The listing builds one solid part. Answer for the finished solid, in the listing's coordinates (mm). A direction names the side the tool comes from. Give positions to 0.01 mm unless a question says otherwise; leave off trailing zeros. Write each loop counter-clockwise with the first axis right and the second up, starting at its lowest first coordinate (ties: lowest second). Pieces come first, ordered by that corner, then holes. Notation, with made-up numbers: (18.5, 26.5) - (49.5, 26.5) arc R17 ccw to (49.5, 33.5) - close; hole circle Ø7 at (-11.5, -19). An arc over 180 degrees is marked (long way). Return JSON: item names as keys, results as strings.
from build123d import *

# Parameters (mm, degrees)
SKETCH_1_W                = 78
SKETCH_1_H                = 15
EXTRUDE_1_DEPTH           = 3
SKETCH_3_R                = 1.5
CUT_EXTRUDE_1_DEPTH       = 3
SKETCH_4_R                = 6
EXTRUDE_2_DEPTH           = 18
SKETCH_5_R                = 4.5
CUT_EXTRUDE_2_DEPTH       = 21
F_2_0MM_2_D               = 3
F_2_0MM_2_DEPTH           = 4.5
F_2_0MM_2_TIP             = 1.5
F_2_0MM_2_ON_FACE_2_D     = 3
F_2_0MM_2_ON_FACE_2_DEPTH = 4.5
F_2_0MM_2_ON_FACE_2_TIP   = 1.5
SKETCH_10_W               = 6
SKETCH_10_H               = 10
CUT_EXTRUDE_3_DEPTH       = 7
SKETCH_13_W               = 19.835687411
SKETCH_13_H               = 21.610205193
CUT_EXTRUDE_4_DEPTH       = 20
SKETCH_14_W               = 11.523038103
SKETCH_14_H               = 10.49031299
EXTRUDE_3_DEPTH           = 3
SKETCH_18_W               = 78
SKETCH_18_H               = 8
EXTRUDE_4_DEPTH           = 3
SKETCH_19_W               = 36.767904102
SKETCH_19_H               = 2.5
EXTRUDE_5_DEPTH           = 12.5
SKETCH_23_R               = 1.65
CUT_EXTRUDE_6_DEPTH       = 12.5
SKETCH_25_W               = 4.236607592
SKETCH_25_H               = 5.36409187
EXTRUDE_7_DEPTH           = 2.5
SKETCH_26_R               = 1.6
CUT_EXTRUDE_7_DEPTH       = 2.5
SKETCH_27_W               = 21.346012392
SKETCH_27_H               = 6.594354882
EXTRUDE_8_DEPTH           = 2.5
SKETCH_28_W               = 36.767231154
SKETCH_28_H               = 5.91819544
EXTRUDE_9_DEPTH           = 2.5
SKETCH_29_W               = 27.660340415
SKETCH_29_H               = 3.5
CUT_EXTRUDE_9_DEPTH       = 2.5
SKETCH_30_W               = 78
SKETCH_30_H               = 8
CUT_EXTRUDE_10_DEPTH      = 100
SKETCH_31_W               = 60.820132647
SKETCH_31_H               = 3
EXTRUDE_10_DEPTH          = 49
SKETCH_32_W               = 48
SKETCH_32_H               = 3.2
CUT_EXTRUDE_11_DEPTH      = 49


with BuildPart() as part:
    # 草图1 → 凸台-拉伸1 (new body)
    with BuildSketch(Plane(origin=(0, 0, 0), x_dir=(1, 0, 0), z_dir=(0, 1, 0))):
        Rectangle(SKETCH_1_W, SKETCH_1_H)
    extrude(amount=EXTRUDE_1_DEPTH)

    # 草图3 → 切除-拉伸1 (cut)
    with BuildSketch(Plane(origin=(0, 3, 0), x_dir=(1, 0, 0), z_dir=(0, 1, 0))):
        with Locations(Location((-34.76, -1.72, 0), (0, 0, 270))):
            Circle(SKETCH_3_R)
        with Locations(Location((-24.35, 4.1, 0), (0, 0, 270))):
            Circle(SKETCH_3_R)
        with Locations(Location((31.56, 4.221692081, 0), (0, 0, 270))):
            Circle(SKETCH_3_R)
        with Locations(Location((7.56, 4.221692081, 0), (0, 0, 270))):
            Circle(SKETCH_3_R)
    extrude(amount=-CUT_EXTRUDE_1_DEPTH, mode=Mode.SUBTRACT)

    # 草图4 → 凸台-拉伸2 (add)
    with BuildSketch(Plane(origin=(0, 3, 0), x_dir=(1, 0, 0), z_dir=(0, 1, 0))):
        with Locations(Location((-3, -1.234165229, 0), (0, 0, 270))):
            Circle(SKETCH_4_R)
    extrude(amount=EXTRUDE_2_DEPTH)

    # 草图5 → 切除-拉伸2 (cut)
    with BuildSketch(Plane(origin=(0, 21, 0), x_dir=(1, 0, 0), z_dir=(0, 1, 0))):
        with Locations(Location((-3, -1.234165229, 0), (0, 0, 270))):
            Circle(SKETCH_5_R)
    extrude(amount=-CUT_EXTRUDE_2_DEPTH, mode=Mode.SUBTRACT)

    # Ø2.0mm 暗销孔2
    with Locations(Plane(origin=(-7.901331048, 17.342107422, 4.694938836), x_dir=(-0.576795601176, 0, -0.816888507977), z_dir=(-0.816888507977, 0, 0.576795601176))):
        with Locations((0, 0)):
            Hole(F_2_0MM_2_D / 2, depth=F_2_0MM_2_DEPTH)
            with Locations((0, 0, -(F_2_0MM_2_DEPTH + F_2_0MM_2_TIP / 2))):  # 90° drill point
                Cone(0, F_2_0MM_2_D / 2, F_2_0MM_2_TIP, mode=Mode.SUBTRACT)

    # Ø2.0mm 暗销孔2 on face 2
    with Locations(Plane(origin=(1.071764877, 17.164817099, 5.641061052), x_dir=(0.734483043181, 0, -0.678627039897), z_dir=(0.678627039897, 0, 0.734483043181))):
        with Locations((0, 0)):
            Hole(F_2_0MM_2_ON_FACE_2_D / 2, depth=F_2_0MM_2_ON_FACE_2_DEPTH)
            with Locations((0, 0, -(F_2_0MM_2_ON_FACE_2_DEPTH + F_2_0MM_2_ON_FACE_2_TIP / 2))):  # 90° drill point
                Cone(0, F_2_0MM_2_ON_FACE_2_D / 2, F_2_0MM_2_ON_FACE_2_TIP, mode=Mode.SUBTRACT)

    # 草图10 → 切除-拉伸3 (cut)
    with BuildSketch(Plane(origin=(0, 0, -7.5), x_dir=(-1, 0, 0), z_dir=(0, 0, -1))):
        with Locations((3, 8)):
            Rectangle(SKETCH_10_W, SKETCH_10_H)
    extrude(amount=-CUT_EXTRUDE_3_DEPTH, mode=Mode.SUBTRACT)

    # 草图13 → 切除-拉伸4 (cut)
    with BuildSketch(Plane(origin=(0, 0, -7.5), x_dir=(-1, 0, 0), z_dir=(0, 0, -1))):
        with Locations((3.314421038, 13.805102597)):
            Rectangle(SKETCH_13_W, SKETCH_13_H)
    extrude(amount=-CUT_EXTRUDE_4_DEPTH, mode=Mode.SUBTRACT)

    # 草图14 → 凸台-拉伸3 (add)
    with BuildSketch(Plane(origin=(0, 3, 0), x_dir=(1, 0, 0), z_dir=(0, 1, 0))):
        with Locations((-2.989467433, -1.263493391)):
            Rectangle(SKETCH_14_W, SKETCH_14_H)
    extrude(amount=-EXTRUDE_3_DEPTH)

    # 草图18 → 凸台-拉伸4 (add)
    with BuildSketch(Plane.XZ):
        with Locations((0, 11.5)):
            Rectangle(SKETCH_18_W, SKETCH_18_H)
    extrude(amount=-EXTRUDE_4_DEPTH)

    # 草图19 → 凸台-拉伸5 (add)
    with BuildSketch(Plane.XZ):
        with Locations((0.839237194, 14.25)):
            Rectangle(SKETCH_19_W, SKETCH_19_H)
    extrude(amount=EXTRUDE_5_DEPTH)

    # 草图23 → 切除-拉伸6 (cut)
    with BuildSketch(Plane(origin=(0, 0, 13), x_dir=(-1, 0, 0), z_dir=(0, 0, -1))):
        with Locations((-8.603189245, -6.05592298)):
            Circle(SKETCH_23_R)
        with Locations((2.596810755, -6.05592298)):
            Circle(SKETCH_23_R)
    extrude(amount=-CUT_EXTRUDE_6_DEPTH, mode=Mode.SUBTRACT)

    # 草图25 → 凸台-拉伸7 (add)
    with BuildSketch(Plane(origin=(0, 0, 13), x_dir=(-1, 0, 0), z_dir=(0, 0, -1))):
        with Locations((2.330668631, -6.426480946)):
            Rectangle(SKETCH_25_W, SKETCH_25_H)
    extrude(amount=-EXTRUDE_7_DEPTH)

    # 草图26 → 切除-拉伸7 (cut)
    with BuildSketch(Plane(origin=(0, 0, 13), x_dir=(-1, 0, 0), z_dir=(0, 0, -1))):
        with Locations((4.196810755, -6.05592298)):
            Circle(SKETCH_26_R)
    extrude(amount=-CUT_EXTRUDE_7_DEPTH, mode=Mode.SUBTRACT)

    # 草图27 → 凸台-拉伸8 (add)
    with BuildSketch(Plane(origin=(0, 0, 13), x_dir=(-1, 0, 0), z_dir=(0, 0, -1))):
        with Locations((-2.379316694, -6.691741876)):
            Rectangle(SKETCH_27_W, SKETCH_27_H)
    extrude(amount=-EXTRUDE_8_DEPTH)

    # 草图28 → 凸台-拉伸9 (add)
    with BuildSketch(Plane(origin=(0, 0, 13), x_dir=(-1, 0, 0), z_dir=(0, 0, -1))):
        with Locations((-0.839573668, -15.45909772)):
            Rectangle(SKETCH_28_W, SKETCH_28_H)
    extrude(amount=-EXTRUDE_9_DEPTH)

    # 草图29 → 切除-拉伸9 (cut)
    with BuildSketch(Plane(origin=(0, 0, 13), x_dir=(-1, 0, 0), z_dir=(0, 0, -1))):
        with Locations((-0.633763758, -13.394190827)):
            Rectangle(SKETCH_29_W, SKETCH_29_H)
    extrude(amount=-CUT_EXTRUDE_9_DEPTH, mode=Mode.SUBTRACT)

    # 草图30 → 切除-拉伸10 (cut)
    with BuildSketch(Plane(origin=(0, 3, 0), x_dir=(1, 0, 0), z_dir=(0, 1, 0))):
        with Locations((0, -11.5)):
            Rectangle(SKETCH_30_W, SKETCH_30_H)
    extrude(amount=-CUT_EXTRUDE_10_DEPTH, mode=Mode.SUBTRACT)

    # 草图31 → 凸台-拉伸10 (add)
    with BuildSketch(Plane.XZ):
        with Locations((0.65611444, 6)):
            Rectangle(SKETCH_31_W, SKETCH_31_H)
    extrude(amount=EXTRUDE_10_DEPTH)

    # 草图32 → 切除-拉伸11 (cut)
    with BuildSketch(Plane(origin=(0, 0, 4.5), x_dir=(-1, 0, 0), z_dir=(0, 0, -1))):
        with Locations((-0.175604554, -15.854114518)):
            Rectangle(SKETCH_32_W, SKETCH_32_H)
        with Locations((-0.205191163, -23.054114518)):
            Rectangle(SKETCH_32_W, SKETCH_32_H)
        with Locations((-0.173277927, -30.254114518)):
            Rectangle(SKETCH_32_W, SKETCH_32_H)
        with Locations((-0.15338956, -37.454114518)):
            Rectangle(SKETCH_32_W, SKETCH_32_H)
        with Locations((-0.189333293, -44.654114518)):
            Rectangle(SKETCH_32_W, SKETCH_32_H)
        with Locations((-0.276259634, -9.654114518)):
            Rectangle(SKETCH_32_W, SKETCH_32_H)
    extrude(amount=-CUT_EXTRUDE_11_DEPTH, mode=Mode.SUBTRACT)


solid = part.part
Item 1: A cutting plane is placed at B-B on x = -16. Give the number of separate pieces and of enclosed holes in the cut face, then the cut area to 3 significant figures.
Answer below:
{"separate pieces": "7", "enclosed holes": "0", "area": "134 mm²"}
Item 2: Flat-ended cylindrical pins translate along their axes: P1, Ø2.5, axis at y = -29.5, z = 6.5, coming from the +X side; P2, Ø1.5, axis at y = -32, z = 2, coming from the +X side; P3, Ø3, axis at x = -1.5, z = -3, coming from the -Y side; P4, Ø1.5, axis at y = -23, z = 6.5, coming from the -X side. Find the tip coordinate at first contact, or state that the pin passes through.
Answer below:
{"P1": "stops at x = 31.07", "P2": "passes through", "P3": "stops at y = 0", "P4": "stops at x = -29.75"}
Item 3: A cutting plane is placed at A-A on x = -34.76. Determine the outline of the cut face in (y, z).
Answer below:
{"outline": "(0, -7.5) - (3, -7.5) - (3, 0.22) - (0, 0.22) - close; (0, 3.22) - (3, 3.22) - (3, 7.5) - (0, 7.5) - close"}
Item 4: The mould has two halves that part along X. Classify faces 1 (the face through (-23.795, -23, 6)), 2 (the face through (-1, 3, 0)), 3 (the face through (-39, 1, 0)): +X half, -X half, draft (parallel to the pull), parting line (faces both ways), or undercut.
Answer below:
{"face 1": "undercut", "face 2": "draft", "face 3": "-X half"}
Item 5: For faces 4 (the face through (0, -49, 6)), 5 (the face through (1, -11.254, 6)), determine the directions among +Z, -Z, +X, -X, +Y, -Y from which every point of the face is accessible in a straight line to the end or side of a thin tool.
Answer below:
{"face 4": "+Z, -Z, +X, -X, -Y", "face 5": "+Z, -Z"}
Item 6: Consider L1, parallel to X at y = -16, z = 6.75; L2, parallel to X at y = 0.8, z = 1.72; L3, parallel to Y at x = 15, z = -2. Determine where each line is inside the solid, lowest interval first.
Answer below:
{"L1": "x = -29.75 to -23.82, 24.18 to 31.07", "L2": "x = -39 to -36.26, -33.26 to 39", "L3": "y = 0 to 3"}
